The model under review builds one solid part; all positions refer to its coordinate system, in mm. A direction names the side the tool comes from. Give positions to 0.01 mm unless a question says otherwise; leave off trailing zeros. Loops run counter-clockwise (first coordinate to the right, second up) from the corner with the lowest first, then second, coordinate; pieces in that order, holes last. Notation, with made-up numbers: M 3,33 L 50,33 A32 ccw 50,62 Z; hole C 0.25,85.5 d7. An arc over 180 degrees is marked long. Return JSON: item names as keys, results as strings.
```python
from build123d import *

# Parameters (mm, degrees)
SKETCH1_W           = 63.5
SKETCH1_H           = 101.6
BOSS_EXTRUDE1_DEPTH = 38.1
CUT_EXTRUDE1_DEPTH  = 38.1
CUT_EXTRUDE2_DEPTH  = 0.508
SKETCH3_R           = 3.81
SKETCH3_W           = 10.16
SKETCH3_H           = 6.35
SKETCH3_W_2         = 12.7
CUT_EXTRUDE3_DEPTH  = 9.525
SKETCH5_W           = 25.4
SKETCH5_H           = 25.4
CUT_EXTRUDE4_DEPTH  = 1.27


with BuildPart() as part:
    # Sketch1 → Boss-Extrude1 (new body)
    with BuildSketch(Plane(origin=(0, 0, 0), x_dir=(1, 0, 0), z_dir=(0, 1, 0))):
        with Locations((-14.643877551, 9.719387755)):
            Rectangle(SKETCH1_W, SKETCH1_H)
    extrude(amount=BOSS_EXTRUDE1_DEPTH)

    # Sketch2 → Cut-Extrude1 (cut)
    with BuildSketch(Plane.XY.offset(41.080612245)):
        with BuildLine():
            ThreePointArc((-30.043877551, 23.1), (-36.793877551, 16.35), (-30.043877551, 9.6))
            Line((-30.043877551, 9.6), (-30.043877551, 23.1))
        make_face()
        with BuildLine():
            Line((-30.043877551, 23.1), (-30.043877551, 9.6))
            ThreePointArc((-30.043877551, 9.6), (-25.270906778, 11.577029227), (-23.293877551, 16.35))
            ThreePointArc((-23.293877551, 16.35), (-25.270906778, 21.122970773), (-30.043877551, 23.1))
        make_face()
        with BuildLine():
            ThreePointArc((0.756122449, 23.1), (-5.993877551, 16.35), (0.756122449, 9.6))
            Line((0.756122449, 9.6), (0.756122449, 23.1))
        make_face()
        with BuildLine():
            Line((0.756122449, 23.1), (0.756122449, 9.6))
            ThreePointArc((0.756122449, 9.6), (5.529093222, 11.577029227), (7.506122449, 16.35))
            ThreePointArc((7.506122449, 16.35), (5.529093222, 21.122970773), (0.756122449, 23.1))
        make_face()
    extrude(amount=-CUT_EXTRUDE1_DEPTH, mode=Mode.SUBTRACT)

    # Sketch2_3 → Cut-Extrude2 (cut)
    with BuildSketch(Plane.XY.offset(41.080612245)):
        with BuildLine():
            Line((-40.043877551, 26.35), (-40.043877551, 6.35))
            Line((-40.043877551, 6.35), (-30.043877551, 6.35))
            Line((-30.043877551, 6.35), (-30.043877551, 9.6))
            ThreePointArc((-30.043877551, 9.6), (-36.793877551, 16.35), (-30.043877551, 23.1))
            Line((-30.043877551, 23.1), (-30.043877551, 26.35))
            Line((-30.043877551, 26.35), (-40.043877551, 26.35))
        make_face()
        with BuildLine():
            Line((-30.043877551, 9.6), (-30.043877551, 6.35))
            Line((-30.043877551, 6.35), (-20.043877551, 6.35))
            Line((-20.043877551, 6.35), (-20.043877551, 26.35))
            Line((-20.043877551, 26.35), (-30.043877551, 26.35))
            Line((-30.043877551, 26.35), (-30.043877551, 23.1))
            ThreePointArc((-30.043877551, 23.1), (-25.270906778, 21.122970773), (-23.293877551, 16.35))
            ThreePointArc((-23.293877551, 16.35), (-25.270906778, 11.577029227), (-30.043877551, 9.6))
        make_face()
        with BuildLine():
            Line((-9.243877551, 26.35), (-9.243877551, 6.35))
            Line((-9.243877551, 6.35), (0.756122449, 6.35))
            Line((0.756122449, 6.35), (0.756122449, 9.6))
            ThreePointArc((0.756122449, 9.6), (-5.993877551, 16.35), (0.756122449, 23.1))
            Line((0.756122449, 23.1), (0.756122449, 26.35))
            Line((0.756122449, 26.35), (-9.243877551, 26.35))
        make_face()
        with BuildLine():
            Line((0.756122449, 9.6), (0.756122449, 6.35))
            Line((0.756122449, 6.35), (10.756122449, 6.35))
            Line((10.756122449, 6.35), (10.756122449, 26.35))
            Line((10.756122449, 26.35), (0.756122449, 26.35))
            Line((0.756122449, 26.35), (0.756122449, 23.1))
            ThreePointArc((0.756122449, 23.1), (5.529093222, 21.122970773), (7.506122449, 16.35))
            ThreePointArc((7.506122449, 16.35), (5.529093222, 11.577029227), (0.756122449, 9.6))
        make_face()
    extrude(amount=-CUT_EXTRUDE2_DEPTH, mode=Mode.SUBTRACT)

    # Sketch3 → Cut-Extrude3 (cut)
    with BuildSketch(Plane(origin=(0, 0, -60.519387755), x_dir=(-1, 0, 0), z_dir=(0, 0, -1))):
        with Locations((13.373877551, 12.7)):
            Circle(SKETCH3_R)
        with Locations((28.613877551, 22.225)):
            Rectangle(SKETCH3_W, SKETCH3_H)
        with Locations((-4.406122449, 9.525)):
            Rectangle(SKETCH3_W_2, SKETCH3_H)
    extrude(amount=-CUT_EXTRUDE3_DEPTH, mode=Mode.SUBTRACT)

    # Sketch5 → Cut-Extrude4 (cut)
    with BuildSketch(Plane(origin=(0, 38.1, 0), x_dir=(1, 0, 0), z_dir=(0, 1, 0))):
        with Locations((-20.993877551, -15.680612245)):
            Rectangle(SKETCH5_W, SKETCH5_H)
    extrude(amount=-CUT_EXTRUDE4_DEPTH, mode=Mode.SUBTRACT)


solid = part.part
```
1) Wall thickness on L1, parallel to Z at x = -5, y = 18; L2, parallel to X at y = 21.5, z = -54.5; L3, parallel to X at y = 12, z = -58: over which ranges is each line inside the solid? List them lowest first. Write a range as from..to.
From the geometry:
{"L1": "-60.52..2.98", "L2": "-46.39..-33.69, -23.53..17.11", "L3": "-46.39..-17.12, -9.63..-1.94, 10.76..17.11"}
2) Tool access review of faces 1 (the face through (-15, 19, -60.519)), 2 (the face through (-30, 16, 2.981)), 3 (the face through (-9.568, 12.868, -55.824)): name each direction out of +Z, -Z, +X, -X, +Y, -Y from which nothing blocks a thin tool from reaching the whole face with its end or side.
From the geometry:
{"face 1": "-Z, +X, -X, +Y, -Y", "face 2": "+Z", "face 3": "-Z"}
3) The part is to be moulded in two halves that separate along Y. For faces 4 (the face through (-15, 38.1, -10)), 5 (the face through (17.106, 19, -9)), 6 (the face through (-1.944, 9, -56)), say which applies: released by +Y, released by -Y, zero draft, split by the parting line, or undercut.
From the geometry:
{"face 4": "released by +Y", "face 5": "zero draft", "face 6": "undercut"}
4) Consider section B-B on y = 21. Write out the cut boundary in (x, z).
From the geometry:
{"outline": "M -46.39,-60.52 L -33.69,-60.52 L -33.69,-50.99 L -23.53,-50.99 L -23.53,-60.52 L 17.11,-60.52 L 17.11,41.08 L 10.76,41.08 L 10.76,40.57 L 5.65,40.57 L 5.65,2.98 L -4.14,2.98 L -4.14,40.57 L -9.24,40.57 L -9.24,41.08 L -20.04,41.08 L -20.04,40.57 L -25.15,40.57 L -25.15,2.98 L -34.94,2.98 L -34.94,40.57 L -40.04,40.57 L -40.04,41.08 L -46.39,41.08 Z"}
5) Insertion check: pin 1 (1.9 mm diameter, centred on x = -29.5, y = 21.5, fed in from -Z). The pin has a flat end and moves straight along its axis. Give the tip position at first contact, or say it passes through.
From the geometry:
{"pin 1": "z = -50.99"}
6) Consider section A-A on z = -52.5. Write out the cut boundary in (x, y), then the cut area to 3 significant figures.
From the geometry:
{"outline": "M -46.39,0 L 17.11,0 L 17.11,38.1 L -46.39,38.1 Z; hole M -33.69,19.05 L -23.53,19.05 L -23.53,25.4 L -33.69,25.4 Z; hole C -13.37,12.7 d7.62; hole M -1.94,6.35 L 10.76,6.35 L 10.76,12.7 L -1.94,12.7 Z", "area": "2,230 mm²"}
